Could you check a few things on this drawing? It's one solid part, dimensions in mm from its lowest x, y, z. A direction names the side the tool comes from. Round coordinates to 2 decimals unless told otherwise and drop trailing zeros. Write each loop counter-clockwise with the first axis right and the second up, starting at its lowest first coordinate (ties: lowest second). Pieces come first, ordered by that corner, then holes. Notation, with made-up numbers: M 42.5,38.25 L 72.5,38.25 A17 cw 72.5,56.25 Z; hole C 15.5,18.25 d1. An arc over 180 degrees is marked long. One line per item, written item: value. Start each with the question number.
(1) Thinking about a two-plate mould opening in Z: for the marked faces 3, 4 and 5, which applies, released by +Z, released by -Z, zero draft, split by the parting line, or undercut?
(2) I want a section at C-C on y = 1.75. Please give me the cut outline in (x, z).
(3) I'm going to push flat-ended pins straight in: pin 1 Ø1.5 at (x, z) = (25.5, 8.5) entering from +Y; pin 2 Ø1.8 at (x, z) = (18, 1.5) entering from +Y; pin 3 Ø5 at (x, y) = (17.5, 7) entering from -Z; pin 4 Ø0.6 at (y, z) = (12, 40) entering from +X. Where does each tip first touch, or does it pass through?
(4) Which directions (+Z, -Z, +X, -X, +Y, -Y) give clear straight access to the entire face, cutting with the end or side of a thin tool? Please do the marked faces 1 and 2.
(5) If I drill on L1, parallel to Z at x = 23, y = 8.5; L2, parallel to X at y = 1, z = 50; L3, parallel to X at y = 10, z = 58.5, over which ranges is the centre line in solid material (lowest first)?
(6) I want a section at A-A on y = 5.5. Please give me the cut outline in (x, z), and give its area (3 significant figures).
(7) I want a section at B-B on z = 10.5. Please give me the cut outline in (x, y), and give its area (4 significant figures).
(8) I want a section at D-D on x = 10. Please give me the cut outline in (y, z).
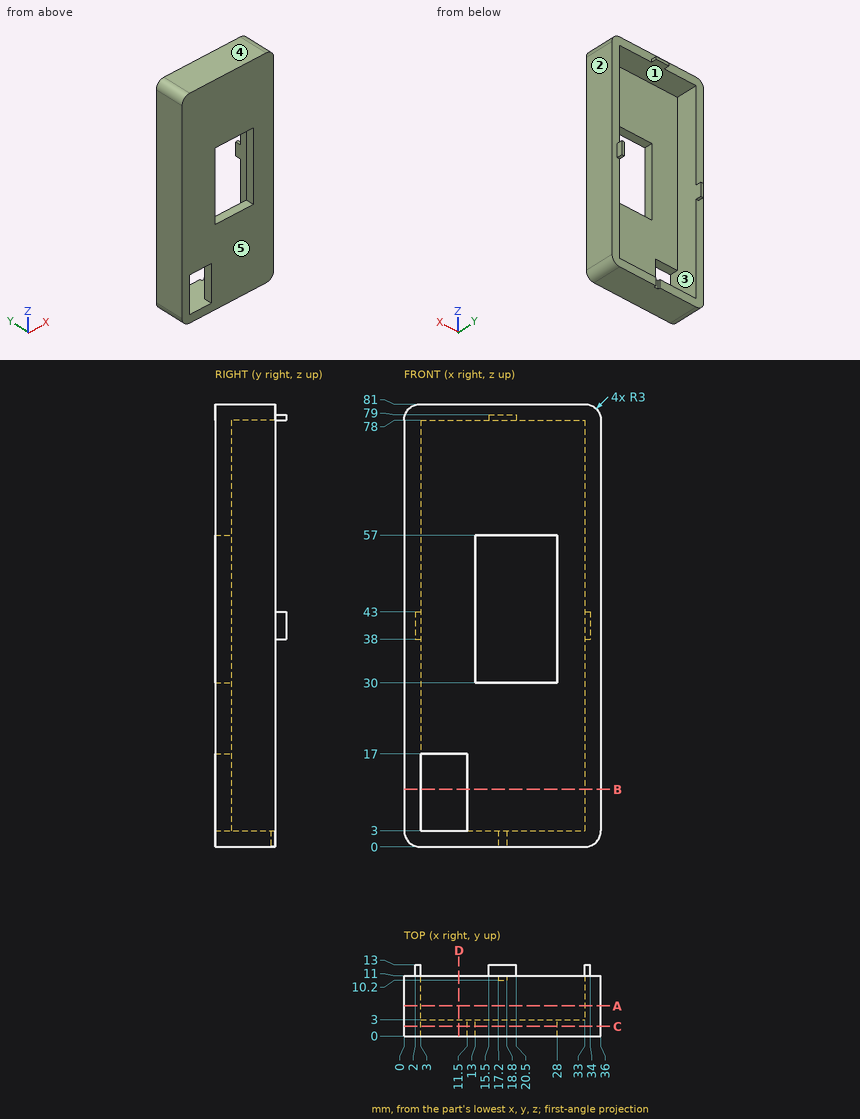
Found:
1. face 3: undercut
1. face 4: released by +Z
1. face 5: zero draft
2. outline: M 0,3 A3 ccw 3,0 L 33,0 A3 ccw 36,3 L 36,78 A3 ccw 33,81 L 3,81 A3 ccw 0,78 Z; hole M 3,3 L 11.5,3 L 11.5,17 L 3,17 Z; hole M 13,30 L 28,30 L 28,57 L 13,57 Z
3. pin 1: stops at y = 3
3. pin 2: stops at y = 11
3. pin 3: stops at z = 0
3. pin 4: stops at x = 34
4. face 1: +Y
4. face 2: +Z, -Z, +X, +Y, -Y
5. L1: z = 0 to 3, 78 to 81
5. L2: x = 0 to 13, 28 to 36
5. L3: x = 0 to 3, 33 to 36
6. outline: M 0,3 A3 ccw 3,0 L 33,0 A3 ccw 36,3 L 36,78 A3 ccw 33,81 L 3,81 A3 ccw 0,78 Z; hole M 3,3 L 33,3 L 33,78 L 3,78 Z
6. area: 658 mm²
7. outline: M 0,0 L 3,0 L 3,11 L 0,11 Z; M 11.5,0 L 36,0 L 36,11 L 33,11 L 33,3 L 11.5,3 Z
7. area: 130.5 mm²
8. outline: M 0,0 L 11,0 L 11,3 L 0,3 Z; M 0,17 L 3,17 L 3,78 L 11,78 L 11,81 L 0,81 Z
